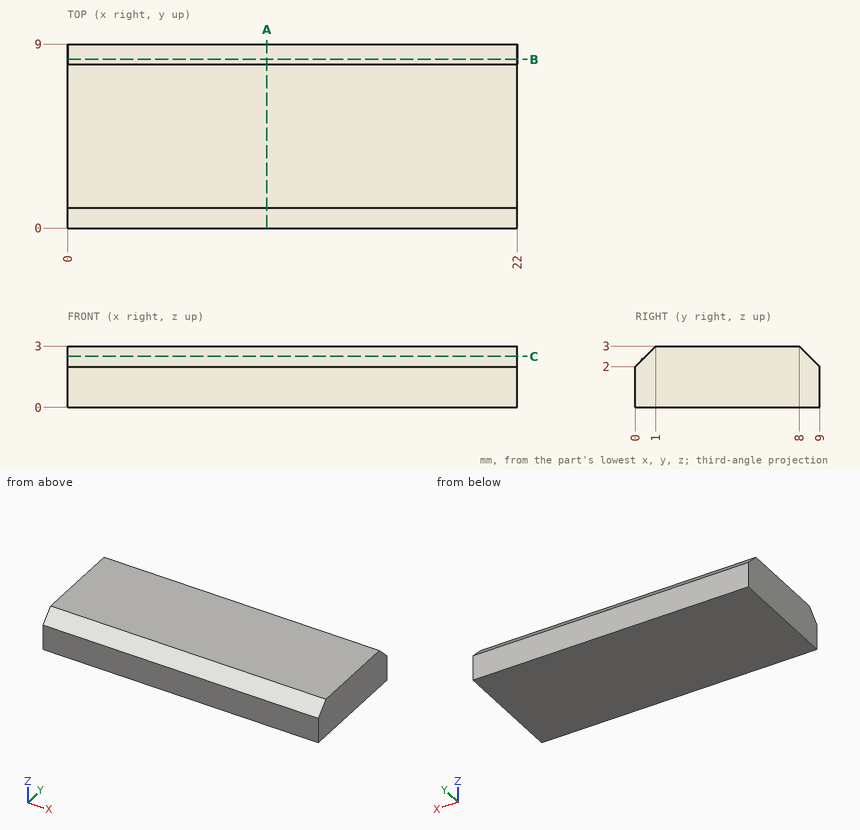
Answer from the drawing. Dimensions are ordinates in mm from the lowest x, y and z of the part. Coordinates: 2 decimals unless noted, no trailing zeros. Write each loop counter-clockwise with the first axis right and the second up, starting at its lowest first coordinate (ties: lowest second). Pieces come first, ordered by that corner, then holes. Notation, with made-up numbers: M 29.5,67.25 L 36.5,67.25 A26 cw 36.5,89.25 Z; hole C -16,10.5 d1. An arc over 180 degrees is marked long. Use one line per item in the form item = value. Start each with the question number.
1. This flat-tipped pin is pushed along its axis until it touches: P1, Ø1, axis at x = 10.5, y = 7, coming from the -Z side. Where does it stop, or does it pass through?
2. Straight lines are drawn through the part: probe 1 along Z at (x, y) = (5.5, 8.75); probe 2 along Y at (x, z) = (11, 2.75); probe 3 along Y at (x, z) = (19.75, 2.4). For each, find the intervals that lie inside material, in ascending order. Write a range as from..to.
3. The part is cut by section C-C (z = 2.5). Give the vertices of the cut face in (x, y).
4. The part is cut by section B-B (y = 8.25). Give the vertices of the cut face in (x, z).
5. The part is cut by section A-A (x = 9.75). Give the vertices of the cut face in (y, z).
Evaluation:
q1.P1 = 0
q2.probe_1 = 0..2.25
q2.probe_2 = 0.75..8.25
q2.probe_3 = 0.4..8.6
q3.outline = M 0,0.5 L 22,0.5 L 22,8.5 L 0,8.5 Z
q4.outline = M 0,0 L 22,0 L 22,2.75 L 0,2.75 Z
q5.outline = M 0,0 L 9,0 L 9,2 L 8,3 L 1,3 L 0,2 Z
